from build123d import *

# Parameters (mm, degrees)
F0_W      = 76.2
F0_H      = 76.2
F1_DEPTH  = 76.2
F3_R      = 14.8282279676
F4_DEPTH  = 101.6
F5_W      = 32.8097548336
F5_H      = 40.4232954606
F6_DEPTH  = 25.4
F7_R      = 12.7
F8_DEPTH  = 88.9
F10_R     = 14.9606
F11_DEPTH = 101.6
F12_W     = 39.3708851188
F12_H     = 42.2465577722
F13_DEPTH = 25.4
F15_DEPTH = 76.2
F17_DEPTH = 25.4
F19_DEPTH = 25.4
F20_R     = 24.146442962
F21_DEPTH = 38.1
F22_W     = 139.7
F22_H     = 114.3
F23_DEPTH = 38.1
F24_W     = 38.1
F24_H     = 38.1
F25_DEPTH = 38.1
F26_W     = 38.1
F26_H     = 38.1
F27_DEPTH = 38.1
F28_R     = 19.05
F29_DEPTH = 139.7
F30_R     = 19.05
F31_DEPTH = 139.7
F32_W     = 63.5
F32_H     = 88.9
F33_DEPTH = 50.8
F34_W     = 63.5
F34_H     = 88.9
F35_DEPTH = 50.8
F36_R     = 20.1986205594
F37_DEPTH = 38.1
F38_W     = 152.4
F38_H     = 76.2
F39_DEPTH = 88.9
F40_R     = 22.1928241729
F41_DEPTH = 12.7
F43_DEPTH = 12.7
F44_R     = 7.7494009563
F45_DEPTH = 12.7
F46_W     = 77.1328099072
F46_H     = 12.1117681265
F47_DEPTH = 5.08


with BuildPart() as f1:
    # F0 (on Front) → F1 (new body)
    with BuildSketch(Plane.XZ):
        with Locations((38.1, 38.1)):
            Rectangle(F0_W, F0_H)
    extrude(amount=F1_DEPTH)

    # F3 (on face) → F4 (join)
    with BuildSketch(Plane.YZ.offset(76.2)):
        with Locations((-35.3661105037, 35.6148853898)):
            Circle(F3_R)
    extrude(amount=F4_DEPTH)

    # F5 (on face) → F6 (join)
    with BuildSketch(Plane.YZ.offset(177.8)):
        with Locations((-34.6139231697, 34.7698931582)):
            Rectangle(F5_W, F5_H)
    extrude(amount=F6_DEPTH)

    # F7 (on face) → F8 (join)
    with BuildSketch(Plane.XZ.offset(51.0188005865)):
        with Locations((190.5, 36.6041734815)):
            Circle(F7_R)
    extrude(amount=F8_DEPTH)

    # F10 (on face) → F11 (join)
    with BuildSketch(Plane(origin=(0, 0, 0), x_dir=(0, -1, 0), z_dir=(-1, 0, 0))):
        with Locations((38.0133911967, 38.1359569728)):
            Circle(F10_R)
    extrude(amount=F11_DEPTH)

    # F12 (on face) → F13 (join)
    with BuildSketch(Plane(origin=(-101.6, 0, 0), x_dir=(0, -1, 0), z_dir=(-1, 0, 0))):
        with Locations((38.3626231924, 38.6948138475)):
            Rectangle(F12_W, F12_H)
    extrude(amount=F13_DEPTH)

    # F14 (on face) → F15 (join)
    with BuildSketch(Plane.XZ.offset(58.0480657518)):
        with BuildLine():
            ThreePointArc((-127, 36.7887159047), (-113.7693257582, 26.1444457534), (-102.2015897118, 38.5758057237))
            ThreePointArc((-102.2015897118, 38.5758057237), (-113.7693257582, 51.0071656939), (-127, 40.3628955426))
            Line((-127, 40.3628955426), (-127, 36.7887159047))
        make_face()
    extrude(amount=F15_DEPTH)

    # F16 (on face) → F17 (join)
    with BuildSketch(Plane.XZ.offset(134.2480657518)):
        Polygon((-102.2015897118, 31.3799439574), (-102.2015897118, 45.77166749), (-114.6651878953, 52.9675292563), (-127.1287860788, 45.77166749), (-127.1287860788, 31.3799439574), (-114.6651878953, 24.1840821911), align=None)
    extrude(amount=F17_DEPTH)

    # F18 (on face) → F19 (join)
    with BuildSketch(Plane.XZ.offset(139.9188005865)):
        Polygon((199.3113872654, 24.8818534128), (205.0575206035, 38.3738986616), (196.246133338, 50.0962187302), (181.6886127346, 48.3264935501), (175.9424793965, 34.8344483013), (184.753866662, 23.1121282327), align=None)
    extrude(amount=F19_DEPTH)

    # F20 (on face) → F21 (join)
    with BuildSketch(Plane(origin=(0, 0, 0), x_dir=(1, 0, 0), z_dir=(0, 0, -1))):
        with Locations((37.9811637104, 38.4700596333)):
            Circle(F20_R)
    extrude(amount=F21_DEPTH)

    # F22 (on face) → F23 (join)
    with BuildSketch(Plane(origin=(0, 0, -38.1), x_dir=(1, 0, 0), z_dir=(0, 0, -1))):
        with Locations((36.0907144785, 36.826572606)):
            Rectangle(F22_W, F22_H)
    extrude(amount=F23_DEPTH)

    # F24 (on face) → F25 (join)
    with BuildSketch(Plane.YZ.offset(105.9407144785)):
        with Locations((-30.6454657137, -57.15)):
            Rectangle(F24_W, F24_H)
    extrude(amount=F25_DEPTH)

    # F26 (on face) → F27 (join)
    with BuildSketch(Plane(origin=(-33.7592855215, 0, 0), x_dir=(0, -1, 0), z_dir=(-1, 0, 0))):
        with Locations((33.1958828002, -57.15)):
            Rectangle(F26_W, F26_H)
    extrude(amount=F27_DEPTH)

    # F28 (on face) → F29 (join)
    with BuildSketch(Plane(origin=(0, 0, -76.2), x_dir=(1, 0, 0), z_dir=(0, 0, -1))):
        with Locations((124.1594851017, 32.0131704211)):
            Circle(F28_R)
    extrude(amount=F29_DEPTH)

    # F30 (on face) → F31 (join)
    with BuildSketch(Plane(origin=(0, 0, -76.2), x_dir=(1, 0, 0), z_dir=(0, 0, -1))):
        with Locations((-51.9242584705, 33.9441895485)):
            Circle(F30_R)
    extrude(amount=F31_DEPTH)

    # F32 (on face) → F33 (join)
    with BuildSketch(Plane(origin=(0, 0, -215.9), x_dir=(1, 0, 0), z_dir=(0, 0, -1))):
        with Locations((-49.5505024791, 33.7955579877)):
            Rectangle(F32_W, F32_H)
    extrude(amount=F33_DEPTH)

    # F34 (on face) → F35 (join)
    with BuildSketch(Plane(origin=(0, 0, -215.9), x_dir=(1, 0, 0), z_dir=(0, 0, -1))):
        with Locations((124.1594851017, 32.0131704211)):
            Rectangle(F34_W, F34_H)
    extrude(amount=F35_DEPTH)

    # F36 (on face) → F37 (join)
    with BuildSketch(Plane.XY.offset(76.2)):
        with Locations((38.3004583418, -37.8415174782)):
            Circle(F36_R)
    extrude(amount=F37_DEPTH)

    # F38 (on face) → F39 (join)
    with BuildSketch(Plane.XY.offset(114.3)):
        with Locations((46.3255597174, -38.1)):
            Rectangle(F38_W, F38_H)
    extrude(amount=F39_DEPTH)

    # F40 (on face) → F41 (join)
    with BuildSketch(Plane.XZ.offset(76.2)):
        with Locations((0, 166.8851673603)):
            Circle(F40_R)
    extrude(amount=F41_DEPTH)

    # F42 (on face) → F43 (join)
    with BuildSketch(Plane.XZ.offset(76.2)):
        Polygon((88.0750278551, 145.0237293252), (104.6800156515, 171.2694208614), (84.8501031118, 195.172067422), (55.9895553719, 183.6990238813), (57.9826684744, 152.7056464582), align=None)
    extrude(amount=F43_DEPTH)

    # F44 (on face) → F45 (join)
    with BuildSketch(Plane(origin=(-127.1287860788, 0, 0), x_dir=(0, -1, 0), z_dir=(-1, 0, 0))):
        with Locations((146.9480657518, 40.6018458307)):
            Circle(F44_R)
    extrude(amount=F45_DEPTH)

    # F46 (on face) → F47 (join)
    with BuildSketch(Plane.XZ.offset(76.2)):
        with Locations((46.0010524839, 127.6153102517)):
            Rectangle(F46_W, F46_H)
    extrude(amount=F47_DEPTH)


solid = f1.part
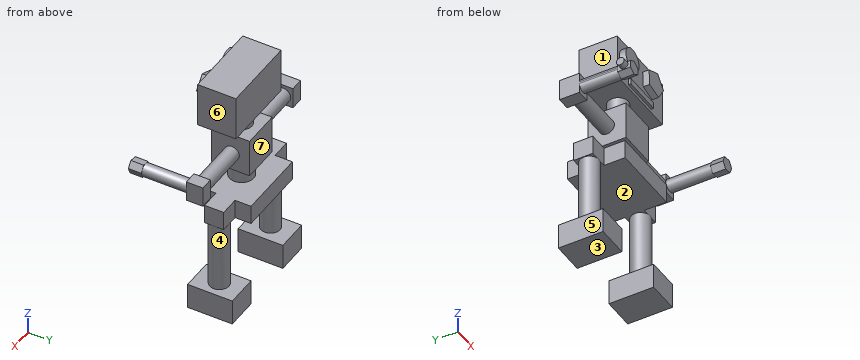
Verification items for the finished model (mm, model axes). Face numbers are marked on the shaded views. A direction names the side the tool comes from. Round coordinates to 2 decimals unless told otherwise and drop trailing zeros. Loops run counter-clockwise (first coordinate to the right, second up) from the corner with the lowest first, then second, coordinate; pieces in that order, holes last. Notation, with made-up numbers: (55, 56.25) - (101, 56.25) arc R25 ccw to (101, 68.25) - close; hole circle Ø11 at (10.25, 80). An arc over 180 degrees is marked (long way). Answer in a Markdown table with one row per item. Add a question column.
Q1. Section check D-D on y = -119. Enter the section's corners in (x, z), plus the area to 3 significant figures.
Q2. Section check B-B on z = 70.5. Enter the section's corners in (x, y).
Q3. Section check A-A on x = -7. Enter the section's corners in (y, z).
Q4. Release check for a two-part mould opening along X. For the marked faces 1, 2 and 3 record: pulls with the +X half, pulls with the -X half, needs draft (parallel to the pull), parting line crosses it, or undercut.
Q5. Section check C-C on z = -101. Enter the section's corners in (x, y), plus the area to 3 significant figures.
Q6. Material ranges on line 1 (Z direction, x = 88, y = -57); line 2 (Z direction, x = -57, y = -17); line 3 (Z direction, x = 35.5, y = -36), recorded low to high.
Q7. Tool access check on the marked faces 4, 5, 6 and 7. Record the directions out of +Z, -Z, +X, -X, +Y, -Y that give a thin tool (end or side, any length) a straight path to the whole face; none if there is none.
Q8. Gauge pin test, flat ends, axial feed: pin 1 (24.5 mm diameter, centred on x = 78.5, z = 159, fed in from -Y); pin 2 (15 mm diameter, centred on y = -13.5, z = -244.5, fed in from -X); pin 3 (8 mm diameter, centred on y = -47, z = -164, fed in from +X). Record the tip position at first contact, or that the pin passes through.
Found:
| question | item | result |
|---|---|---|
| 1 | outline | (-127, 36.79) arc R12.46 ccw (long way) to (-127, 40.36) - close; circle Ø25.4 at (190.5, 36.6) |
| 1 | area | 994 mm² |
| 2 | outline | (0, -76.2) - (76.2, -76.2) - (76.2, 0) - (0, 0) - close |
| 3 | outline | (-93.98, -76.2) - (20.32, -76.2) - (20.32, -38.1) - (-93.98, -38.1) - close; (-88.9, 145.83) - (-76.2, 145.83) - (-76.2, 114.3) - (0, 114.3) - (0, 203.2) - (-76.2, 203.2) - (-76.2, 187.95) - (-88.9, 187.95) - close; circle Ø29.92 at (-38.01, 38.14) |
| 4 | face 1 | pulls with the -X half |
| 4 | face 2 | undercut |
| 4 | face 3 | needs draft |
| 5 | outline | circle Ø38.1 at (-51.92, -33.94); circle Ø38.1 at (124.16, -32.01) |
| 5 | area | 2,280 mm² |
| 6 | line 1 | z = -76.2 to -38.1, 114.3 to 203.2 |
| 6 | line 2 | z = -266.7 to -38.1 |
| 6 | line 3 | z = -76.2 to 203.2 |
| 7 | face 4 | none |
| 7 | face 5 | -Z, -X, +Y, -Y |
| 7 | face 6 | +Z, +X, +Y, -Y |
| 7 | face 7 | +Z, +X, -X, +Y |
| 8 | pin 1 | stops at y = -88.9 |
| 8 | pin 2 | stops at x = -81.3 |
| 8 | pin 3 | stops at x = 139.72 |
